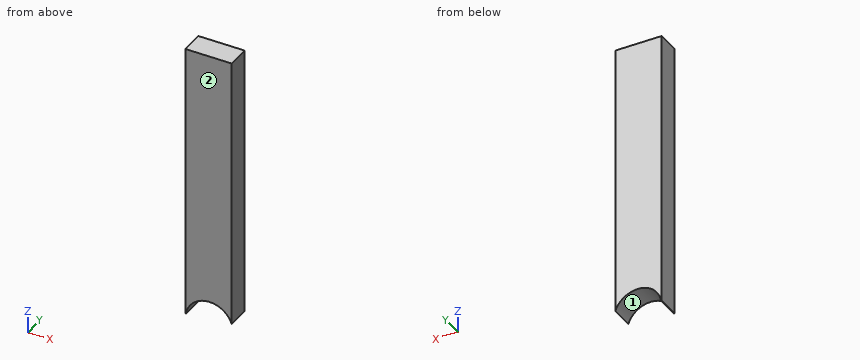
from build123d import *

# Parameters (mm, degrees)
F0_W     = 12.7
F0_H     = 76.2
F1_DEPTH = 6.35
F2_R     = 6.475828
F3_DEPTH = 12.7


with BuildPart() as f1:
    # F0 (on Front) → F1 (new body)
    with BuildSketch(Plane.XZ):
        with Locations((-21.859534, 5.321618)):
            Rectangle(F0_W, F0_H)
    extrude(amount=F1_DEPTH)

    # F2 (on Front) → F3 (cut, symmetric)
    with BuildSketch(Plane.XZ):
        with Locations((-21.623934, -33.730884)):
            Circle(F2_R)
    extrude(amount=F3_DEPTH, both=True, mode=Mode.SUBTRACT)


solid = f1.part
The model under review builds one solid part; all positions refer to its coordinate system, in mm. Face numbers are marked on the shaded views. Coordinates: 2 decimals unless noted, no trailing zeros. Write each loop counter-clockwise with the first axis right and the second up, starting at its lowest first coordinate (ties: lowest second). Pieces come first, ordered by that corner, then holes. Notation, with made-up numbers: M -7,32.5 L -2,32.5 A10 ccw -2,47.5 Z; hole C 15.5,-9.5 d9. An arc over 180 degrees is marked long. Put each result on its own line as item: value.
1) Add section A-A on y = -1.25. Give the boundary of the cut face in (x, z), then the cut area to 3 significant figures.
Computed:
outline: M -28.21,-32.78 L -28.03,-32.78 A6.48 cw -15.51,-31.6 L -15.51,43.42 L -28.21,43.42 Z
area: 914 mm2
2) Wall thickness on probe 1 along Z at (x, y) = (-22, -3); probe 2 along Z at (x, y) = (-25, -0.5): over which ranges is each line inside the solid? List them lowest first. Write a range as [from, to].
Computed:
probe 1: z = [-27.27, 43.42]
probe 2: z = [-28.2, 43.42]
3) Draft analysis for pull direction X (two halves, no side actions). For the marked faces 1 and 2, state which applies: released by +X, released by -X, zero draft, split by the parting line, or undercut.
Computed:
face 1: undercut
face 2: zero draft
4) Add section B-B on x = -18.5. Give the boundary of the cut face in (y, z), then the cut area to 3 significant figures.
Computed:
outline: M -6.35,-28.06 L 0,-28.06 L 0,43.42 L -6.35,43.42 Z
area: 454 mm2
5) Add section C-C on x = -22.25. Give the boundary of the cut face in (y, z), then the cut area to 3 significant figures.
Computed:
outline: M -6.35,-27.29 L 0,-27.29 L 0,43.42 L -6.35,43.42 Z
area: 449 mm2
